Check sheet for the modelled part. Datum: model origin and axes. Units: mm. Face numbers are marked on the shaded views. A direction names the side the tool comes from. Round coordinates to 2 decimals unless told otherwise and drop trailing zeros. Loops run counter-clockwise (first coordinate to the right, second up) from the corner with the lowest first, then second, coordinate; pieces in that order, holes last. Notation, with made-up numbers: (-12.5, 13.5) -> (14.5, 13.5) arc R23 ccw to (14.5, 35.5) -> close; hole circle Ø11 at (86, 26). An arc over 180 degrees is marked (long way). Use one line per item in the form item = value. Start each with the question number.
(1) Sectioned sample at C-C (z = 22.5). Record the cut outline in (x, y), and give its area (3 significant figures).
(2) Set-up check for the marked faces 1 and 2: record each of +Z, -Z, +X, -X, +Y, -Y from which the full face is reachable in a straight line by a thin tool's end or side.
(3) Go/stop test with flat-tipped pins: pin 1 (12 mm diameter, centred on y = -17, z = -0.5, fed in from -X); pin 2 (1.7 mm diameter, centred on x = -13, y = -23, fed in from +Z); pin 3 (1.5 mm diameter, centred on x = 27.5, z = -5.5, fed in from +Y) (3 decimals). Record where each tip stops, or that it passes through.
(4) Sectioned sample at A-A (z = 17). Record the cut outline in (x, y).
(5) Material ranges on probe 1 along Y at (x, z) = (0.5, 13); probe 2 along Y at (x, z) = (0, -3.8); probe 3 along Z at (x, y) = (-17, -10), recorded low to high. Write a range as [from, to].
(6) Draft check along Y on the marked faces 3, 4 and 5. Enter one of: released by +Y, released by -Y, zero draft, split by the parting line, or undercut.
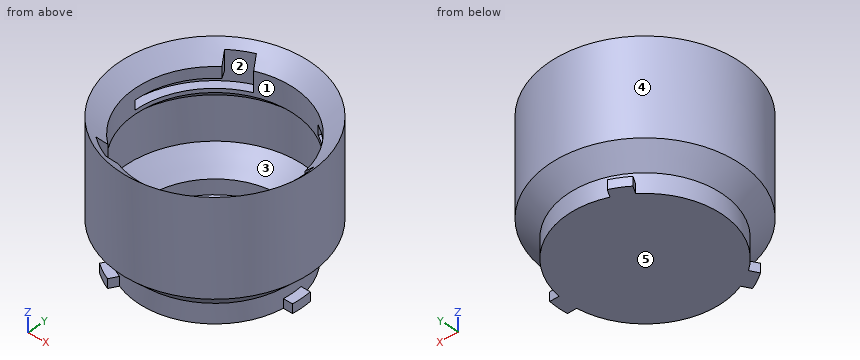
from build123d import *

# Parameters (mm, degrees)
F0_R             = 25.4
F1_DEPTH         = 6.35
F3_DEPTH         = 3
F4_R             = 22.4
F5_DEPTH         = 3.35
F6_R             = 31.4
F6_R_2           = 22.4
F7_DEPTH         = 31.75
F9_DEPTH         = 6.35
F10_R            = 26.15
F11_DEPTH        = 28
F12_W            = 10.4017283041
F12_H            = 3.1
F14_COPIES_COUNT = 3
F16_SIZE         = 5.99999
F17_R            = 31.4
F17_R_2          = 26.15
F18_DEPTH        = 6.35
F20_DEPTH        = 25


# Not quite as in the source:
# - a fillet or chamfer that OpenCascade refuses, or shapes differently, is made with other operations: its cross-section is extruded or revolved along the edge and cut away or added
# - a fillet or chamfer is up to 0.001 mm smaller than in the source, because OpenCascade refuses the exact size
# - a pattern or mirror of a feature is missing from the dataset's text; its kind, count and spacing are read off the source's solid


with BuildPart() as f1:
    # F0 (on Top) → F1 (new body)
    with BuildSketch(Plane.XY):
        Circle(F0_R)
    extrude(amount=-F1_DEPTH)

    # F2 (on face) → F3 (join)
    with BuildSketch(Plane(origin=(0, 0, -6.35), x_dir=(1, 0, 0), z_dir=(0, 0, -1))):
        with BuildLine():
            ThreePointArc((28.2219661788, -3.175), (28.4, 0), (28.2219661788, 3.175))
            Line((28.2219661788, 3.175), (22.4, 3.175))
            Line((22.4, 3.175), (22.4, -3.175))
            Line((22.4, -3.175), (28.2219661788, -3.175))
        make_face()
        with BuildLine():
            Line((-8.450369343, 20.9864690448), (-11.3613524324, 26.0284396556))
            ThreePointArc((-11.3613524324, 26.0284396556), (-14.2, 24.5951214675), (-16.8606137464, 22.8534396556))
            Line((-16.8606137464, 22.8534396556), (-13.949630657, 17.8114690448))
            Line((-13.949630657, 17.8114690448), (-8.450369343, 20.9864690448))
        make_face()
        with BuildLine():
            Line((-13.949630657, -17.8114690448), (-16.8606137464, -22.8534396556))
            ThreePointArc((-16.8606137464, -22.8534396556), (-14.2, -24.5951214675), (-11.3613524324, -26.0284396556))
            Line((-11.3613524324, -26.0284396556), (-8.450369343, -20.9864690448))
            Line((-8.450369343, -20.9864690448), (-13.949630657, -17.8114690448))
        make_face()
    extrude(amount=-F3_DEPTH)

    # F4 (on face) → F5 (cut, through all)
    with BuildSketch(Plane.XY):
        Circle(F4_R)
    extrude(amount=-F5_DEPTH, mode=Mode.SUBTRACT)

    # F6 (on face) → F7 (join)
    with BuildSketch(Plane.XY):
        Circle(F6_R)
        Circle(F6_R_2, mode=Mode.SUBTRACT)
    extrude(amount=F7_DEPTH)

    # F8 (on face) → F9 (cut)
    with BuildSketch(Plane.XY.offset(31.75)):
        with BuildLine():
            Line((17.4498241395, -3.925), (28.8845438773, -3.925))
            ThreePointArc((28.8845438773, -3.925), (29.15, 0), (28.8845438773, 3.925))
            Line((28.8845438773, 3.925), (17.4498241395, 3.925))
            Line((17.4498241395, 3.925), (17.4498241395, 0))
            Line((17.4498241395, 0), (17.4498241395, -3.925))
        make_face()
        with BuildLine():
            Line((-5.3257623599, 17.0744909964), (-11.0431222288, 26.9772487745))
            ThreePointArc((-11.0431222288, 26.9772487745), (-14.575, 25.2446405203), (-17.8414216485, 23.0522487745))
            Line((-17.8414216485, 23.0522487745), (-12.1240617796, 13.1494909964))
            Line((-12.1240617796, 13.1494909964), (-8.7249120697, 15.1119909964))
            Line((-8.7249120697, 15.1119909964), (-5.3257623599, 17.0744909964))
        make_face()
        with BuildLine():
            Line((-12.1240617796, -13.1494909964), (-17.8414216485, -23.0522487745))
            ThreePointArc((-17.8414216485, -23.0522487745), (-14.575, -25.2446405203), (-11.0431222288, -26.9772487745))
            Line((-11.0431222288, -26.9772487745), (-5.3257623599, -17.0744909964))
            Line((-5.3257623599, -17.0744909964), (-8.7249120697, -15.1119909964))
            Line((-8.7249120697, -15.1119909964), (-12.1240617796, -13.1494909964))
        make_face()
    extrude(amount=-F9_DEPTH, mode=Mode.SUBTRACT)

    # F10 (on face) → F11 (cut)
    with BuildSketch(Plane.XY.offset(31.75)):
        Circle(F10_R)
    extrude(amount=-F11_DEPTH, mode=Mode.SUBTRACT)

    # F14: sweep along a path in F13
    with BuildLine(Plane.XY.offset(31.75)) as f14_path:
        ThreePointArc((37.4274057464, 0), (32.4130841741, 18.7137028732), (18.7137028732, 32.4130841741))
    # F12 (on Front) → F14 (sweep, cut)
    with BuildSketch(Plane.XZ):
        with Locations((23.949135848, 26.95)):
            Rectangle(F12_W, F12_H)
    f14 = sweep(path=f14_path.line, mode=Mode.SUBTRACT)

    # F14_copies: F14 ×3 about axis
    f14_copies_axis = Axis((0, 0, 0), (0, 0, 1))
    for i in range(1, F14_COPIES_COUNT):
        add(f14.rotate(f14_copies_axis, i * 360 / F14_COPIES_COUNT), mode=Mode.SUBTRACT)

    # F16 (size 6 in the source; OpenCascade refuses exactly that, so slightly less here)
    f16_edges = [f1.edges().sort_by_distance(p)[0] for p in [
        (-31.4, 0, 0),
    ]]
    chamfer(f16_edges, length=F16_SIZE)

    # F17 (on face) → F18 (join)
    with BuildSketch(Plane.XY.offset(31.75)):
        Circle(F17_R)
        Circle(F17_R_2, mode=Mode.SUBTRACT)
    extrude(amount=F18_DEPTH)

    # F19: chamfer of 6 on 1 edges, made by hand

    # F19_s1 → F19_t2 (revolve, cut)
    with BuildSketch(Plane.XZ):
        Polygon((32.15, 38.1), (26.15, 32.1), (26.15, 38.1), align=None)
    revolve(axis=Axis((0, 0, 38.1), (0, 0, 1)), mode=Mode.SUBTRACT)

    # F8 (on face) → F20 (cut)
    with BuildSketch(Plane.XY.offset(31.75)):
        with BuildLine():
            Line((17.4498241395, -3.925), (28.8845438773, -3.925))
            ThreePointArc((28.8845438773, -3.925), (29.15, 0), (28.8845438773, 3.925))
            Line((28.8845438773, 3.925), (17.4498241395, 3.925))
            Line((17.4498241395, 3.925), (17.4498241395, 0))
            Line((17.4498241395, 0), (17.4498241395, -3.925))
        make_face()
        with BuildLine():
            Line((-5.3257623599, 17.0744909964), (-11.0431222288, 26.9772487745))
            ThreePointArc((-11.0431222288, 26.9772487745), (-14.575, 25.2446405203), (-17.8414216485, 23.0522487745))
            Line((-17.8414216485, 23.0522487745), (-12.1240617796, 13.1494909964))
            Line((-12.1240617796, 13.1494909964), (-8.7249120697, 15.1119909964))
            Line((-8.7249120697, 15.1119909964), (-5.3257623599, 17.0744909964))
        make_face()
        with BuildLine():
            Line((-12.1240617796, -13.1494909964), (-17.8414216485, -23.0522487745))
            ThreePointArc((-17.8414216485, -23.0522487745), (-14.575, -25.2446405203), (-11.0431222288, -26.9772487745))
            Line((-11.0431222288, -26.9772487745), (-5.3257623599, -17.0744909964))
            Line((-5.3257623599, -17.0744909964), (-8.7249120697, -15.1119909964))
            Line((-8.7249120697, -15.1119909964), (-12.1240617796, -13.1494909964))
        make_face()
    extrude(amount=F20_DEPTH, mode=Mode.SUBTRACT)

    # F21 (on Front) → F22 (revolve, cut)
    with BuildSketch(Plane.XZ):
        Polygon((0, 0), (0, -4.85), (23, -4.85), (23, 0), (29.5, 6.5), (29.5, 20.7537593978), (25.8537593978, 24.4), (0, 24.4), align=None)
    revolve(axis=Axis((0, 0, 37.5208705664), (0, 0, 1)), mode=Mode.SUBTRACT)


solid = f1.part
Checks:
q1.outline = circle Ø62.8 at (0, 0); hole circle Ø55.51 at (0, 0)
q1.area = 678 mm2
q2.face_1 = +Z
q2.face_2 = none
q3.pin_1 = -26.67
q3.pin_2 = 25.4
q3.pin_3 = 3.175
q4.outline = circle Ø62.8 at (0, 0); hole circle Ø59 at (0, 0)
q5.probe_1 = [-31.4, -29.5], [29.5, 31.4]
q5.probe_2 = [-25.4, -23], [23, 25.4]
q5.probe_3 = [-6.35, -4.85]
q6.face_3 = undercut
q6.face_4 = split by the parting line
q6.face_5 = zero draft
